The listing builds one solid part. Answer for the finished solid, in the listing's coordinates (mm). Give positions to 0.01 mm unless a question says otherwise; leave off trailing zeros. Order: outer loops, then holes, each group sorted by start corner. A loop starts at its lowest first (then second) coordinate and runs counter-clockwise, first axis right, second up. Notation, with made-up numbers: (29, -24) - (34, -24) arc R18 cw to (34, 3) - close; hole circle Ø1 at (79, -18.5). An arc over 180 degrees is marked (long way). Answer as a JSON object with one key per item and string values. Group by question number.
Q1. Consider line 1 (Y direction, x = 14.5, z = 2); line 2 (Y direction, x = 11, z = 5.5); line 3 (X direction, y = 58, z = 7.25). Determine where each line is inside the solid, lowest interval first.
Q2. A cutting plane is placed at B-B, the plane z = 0.75. Give the vertices of the cut face in (x, y).
Q3. A cutting plane is placed at A-A, the plane y = 11. Give the vertices of the cut face in (x, z), and give its area (3 significant figures).
Q4. A cutting plane is placed at D-D, the plane x = 3. Give the vertices of the cut face in (y, z), and give its area (3 significant figures).
Q5. A cutting plane is placed at C-C, the plane y = 60. Give the vertices of the cut face in (x, z).
from build123d import *

# Parameters (mm, degrees)
SALIENTE_EXTRUIR2_DEPTH = 8.2


with BuildPart() as part:
    # Croquis1 → Saliente-Extruir2 (new body)
    with BuildSketch(Plane.XY):
        with BuildLine():
            Line((0, 69.4), (0, 34.7))
            Line((0, 34.7), (15.55, 34.7))
            Line((15.55, 34.7), (15.55, 49.4))
            ThreePointArc((15.55, 49.4), (9.55, 55.4), (15.55, 61.4))
            Line((15.55, 61.4), (15.55, 72.55))
            ThreePointArc((15.55, 72.55), (7.617078092, 71.754582753), (0, 69.4))
        make_face()
        with BuildLine():
            Line((15.55, 49.4), (15.55, 34.7))
            Line((15.55, 34.7), (31.1, 34.7))
            Line((31.1, 34.7), (31.1, 69.4))
            ThreePointArc((31.1, 69.4), (23.482921908, 71.754582753), (15.55, 72.55))
            Line((15.55, 72.55), (15.55, 61.4))
            ThreePointArc((15.55, 61.4), (19.792640687, 59.642640687), (21.55, 55.4))
            ThreePointArc((21.55, 55.4), (19.792640687, 51.157359313), (15.55, 49.4))
        make_face()
        with BuildLine():
            Line((0, 34.7), (0, 0))
            ThreePointArc((0, 0), (7.617078092, -2.354582753), (15.55, -3.15))
            Line((15.55, -3.15), (15.55, 8))
            ThreePointArc((15.55, 8), (9.55, 14), (15.55, 20))
            Line((15.55, 20), (15.55, 34.7))
            Line((15.55, 34.7), (0, 34.7))
        make_face()
        with BuildLine():
            Line((15.55, 8), (15.55, -3.15))
            ThreePointArc((15.55, -3.15), (23.482921908, -2.354582753), (31.1, 0))
            Line((31.1, 0), (31.1, 34.7))
            Line((31.1, 34.7), (15.55, 34.7))
            Line((15.55, 34.7), (15.55, 20))
            ThreePointArc((15.55, 20), (19.792640687, 18.242640687), (21.55, 14))
            ThreePointArc((21.55, 14), (19.792640687, 9.757359313), (15.55, 8))
        make_face()
    extrude(amount=SALIENTE_EXTRUIR2_DEPTH)


solid = part.part
Reply:
{
 "1": {"line 1": "y = -3.14 to 8.09, 19.91 to 49.49, 61.31 to 72.54", "line 2": "y = -2.89 to 10.09, 17.91 to 51.49, 59.31 to 72.29", "line 3": "x = 0 to 10.14, 20.96 to 31.1"},
 "2": {"outline": "(0, 0) arc R39.96 ccw to (31.1, 0) - (31.1, 69.4) arc R39.96 ccw to (0, 69.4) - close; hole circle Ø12 at (15.55, 14); hole circle Ø12 at (15.55, 55.4)"},
 "3": {"outline": "(0, 0) - (10.35, 0) - (10.35, 8.2) - (0, 8.2) - close; (20.75, 0) - (31.1, 0) - (31.1, 8.2) - (20.75, 8.2) - close", "area": "170 mm^2"},
 "4": {"outline": "(-1.13, 0) - (70.53, 0) - (70.53, 8.2) - (-1.13, 8.2) - close", "area": "588 mm^2"},
 "5": {"outline": "(0, 0) - (11.7, 0) - (11.7, 8.2) - (0, 8.2) - close; (19.4, 0) - (31.1, 0) - (31.1, 8.2) - (19.4, 8.2) - close"}
}
